CAD build for the part. Positions are in the model's coordinates, mm. A direction names the side the tool comes from. Give positions to 0.01 mm unless a question says otherwise; leave off trailing zeros. Write each loop counter-clockwise with the first axis right and the second up, starting at its lowest first coordinate (ties: lowest second). Pieces come first, ordered by that corner, then holes. Notation, with made-up numbers: M -9,26 L 40,26 A7 ccw 40,30 Z; hole C -10.5,-38.75 d11. An arc over 180 degrees is marked long. One line per question, with ' | ' between items. Start each with the question number.
1. Which spindle directions (+Z, -Z, +X, -X, +Y, -Y) get a long thin tool onto all of the face, cutting with end or side? Do faces 1 (the face through (12, 1.4, 2)), 2 (the face through (-9.2, 0, 2)), 3 (the face through (0, -9.2, 2)), 4 (the face through (-8, 15, 1)). Say none if no direction does.
2. Cut at B-B, the plane z = 0.6. Write the cut outline in (x, y).
3. Cut at A-A, the plane x = 12.75. Write the cut outline in (y, z).
4. Wall check: L1, parallel to Y at x = 12, z = 0.4; L2, parallel to X at y = 1.25, z = 1. Give the ranges that are in metal, low to high.
5. Cut at C-C, the plane y = 0.75. Write the cut outline in (x, z), then the cut area to 3 significant figures.
6. Pull direction Y, two halves, no side cores. Call faces 5 (the face through (0, 9.2, 2)), 6 (the face through (-12, 1.4, 2)), 7 (the face through (15, -8, 1)): released by +Y, released by -Y, zero draft, split by the parting line, or undercut.
7. Flat gauge pins, fed straight in: pin 1 (1.4 mm diameter, centred on x = 0, z = 2, fed in from -Y); pin 2 (0.8 mm diameter, centred on y = 0, z = 1, fed in from +X); pin 3 (0.8 mm diameter, centred on y = -0.5, z = 2, fed in from -X). Where does each tip first touch, or does it go through?
```python
from build123d import *

# Parameters (mm, degrees)
SKETCH1_W               = 30
SKETCH1_H               = 30
BOSS_EXTRUDE1_DEPTH     = 3
SKETCH2_W               = 2.8
SKETCH2_H               = 5.8
SKETCH2_W_2             = 5.8
SKETCH2_H_2             = 2.8
CUT_EXTRUDE1_DEPTH      = 1
CUT_EXTRUDE1_DEPTH_BACK = 4


with BuildPart() as part:
    # Sketch1 → Boss-Extrude1 (new body)
    with BuildSketch(Plane.XY):
        Rectangle(SKETCH1_W, SKETCH1_H)
    extrude(amount=BOSS_EXTRUDE1_DEPTH)

    # Sketch2 → Cut-Extrude1 (cut, two sides)
    with BuildSketch(Plane.XY.offset(3)) as cut_extrude1_sk:
        with Locations((0, 12.1)):
            Rectangle(SKETCH2_W, SKETCH2_H)
        with Locations((0, -12.1)):
            Rectangle(SKETCH2_W, SKETCH2_H)
        with Locations((-12.1, 0)):
            Rectangle(SKETCH2_W_2, SKETCH2_H_2)
        with Locations((12.1, 0)):
            Rectangle(SKETCH2_W_2, SKETCH2_H_2)
    extrude(amount=CUT_EXTRUDE1_DEPTH, mode=Mode.SUBTRACT)
    extrude(cut_extrude1_sk.sketch, amount=-CUT_EXTRUDE1_DEPTH_BACK, mode=Mode.SUBTRACT)


solid = part.part
```
Here are the results:
1) face 1: +Z, -Z, +X | face 2: +Z, -Z, -X | face 3: +Z, -Z, -Y | face 4: +Z, -Z, +X, -X, +Y
2) outline: M -15,-15 L -1.4,-15 L -1.4,-9.2 L 1.4,-9.2 L 1.4,-15 L 15,-15 L 15,-1.4 L 9.2,-1.4 L 9.2,1.4 L 15,1.4 L 15,15 L 1.4,15 L 1.4,9.2 L -1.4,9.2 L -1.4,15 L -15,15 L -15,1.4 L -9.2,1.4 L -9.2,-1.4 L -15,-1.4 Z
3) outline: M -15,0 L -1.4,0 L -1.4,3 L -15,3 Z; M 1.4,0 L 15,0 L 15,3 L 1.4,3 Z
4) L1: -15 to -1.4, 1.4 to 15 | L2: -9.2 to 9.2
5) outline: M -9.2,0 L 9.2,0 L 9.2,3 L -9.2,3 Z | area: 55.2 mm^2
6) face 5: released by +Y | face 6: undercut | face 7: zero draft
7) pin 1: y = -9.2 | pin 2: x = 9.2 | pin 3: x = -9.2
